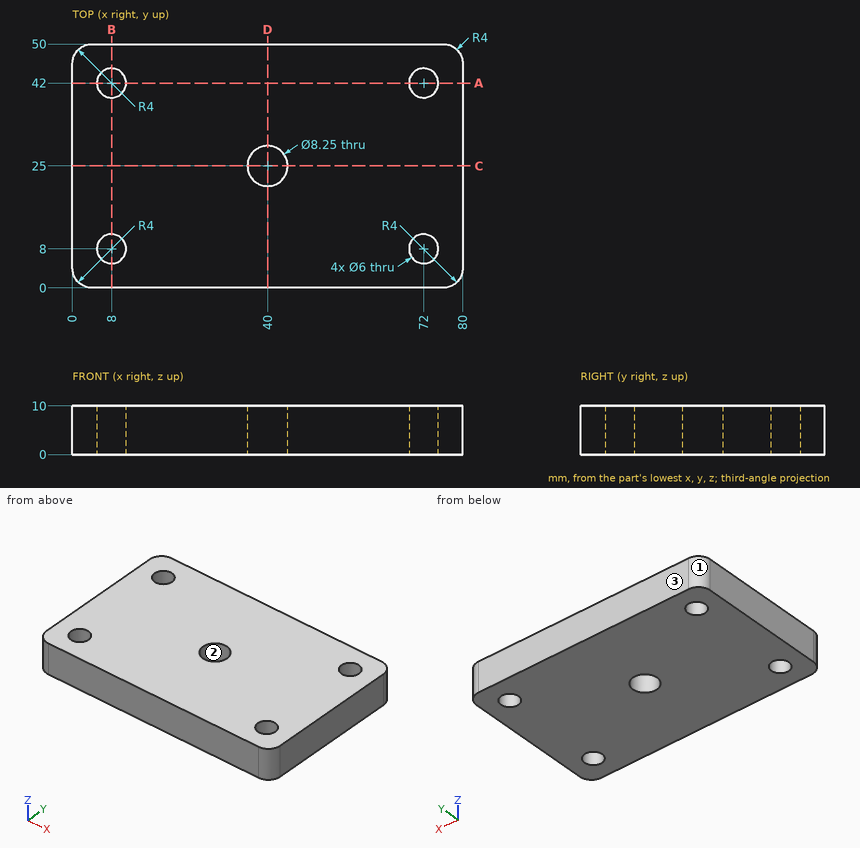
The drawing under review shows one solid part. Ordinate dimensions are in mm from its lowest x, y, z. Round coordinates to 2 decimals unless told otherwise and drop trailing zeros. Order: outer loops, then holes, each group sorted by start corner. A loop starts at its lowest first (then second) coordinate and runs counter-clockwise, first axis right, second up. Notation, with made-up numbers: M 12.5,56 L 68.5,56 A16 ccw 68.5,67 Z; hole C 23,71 d4. An arc over 180 degrees is marked long. Answer as CSV lines item,"result". Start each with the question number.
1) Wall thickness on line 1 along Y through (x, z) = (72, 7.75); line 2 along Y through (x, z) = (40, 7) (3 decimals); line 3 along X through (y, z) = (9, 6): over which ranges is each line inside the solid? List them lowest first. Write a range as [from, to].
2) Add section A-A (y = 42). Give the boundary of the cut face in (x, z), then the cut area to 3 significant figures.
3) For pin 1 Ø8 at (x, y) = (8, 42) entering from -Z; pin 2 Ø5 at (x, y) = (8, 8) entering from -Z, all flat-tipped, find the tip position at first contact; note any pin that passes through.
4) Add section D-D (x = 40). Give the boundary of the cut face in (y, z) (3 decimals).
5) Add section C-C (y = 25). Give the boundary of the cut face in (x, z) (3 decimals).
6) The part is to be moulded in two halves that separate along X. For the marked faces 1, 2 and 3, say which applies: +X half, -X half, draft (parallel to the pull), parting line (faces both ways), or undercut.
7) Add section B-B (x = 8). Give the boundary of the cut face in (y, z).
Resolved:
1,line 1,"[0, 5], [11, 39], [45, 50]"
1,line 2,"[0, 20.875], [29.125, 50]"
1,line 3,"[0, 5.17], [10.83, 69.17], [74.83, 80]"
2,outline,"M 0,0 L 5,0 L 5,10 L 0,10 Z; M 11,0 L 69,0 L 69,10 L 11,10 Z; M 75,0 L 80,0 L 80,10 L 75,10 Z"
2,area,"680 mm^2"
3,pin 1,"z = 0"
3,pin 2,"through"
4,outline,"M 0,0 L 20.875,0 L 20.875,10 L 0,10 Z; M 29.125,0 L 50,0 L 50,10 L 29.125,10 Z"
5,outline,"M 0,0 L 35.875,0 L 35.875,10 L 0,10 Z; M 44.125,0 L 80,0 L 80,10 L 44.125,10 Z"
6,face 1,"-X half"
6,face 2,"undercut"
6,face 3,"draft"
7,outline,"M 0,0 L 5,0 L 5,10 L 0,10 Z; M 11,0 L 39,0 L 39,10 L 11,10 Z; M 45,0 L 50,0 L 50,10 L 45,10 Z"
